Geometry check sheet. Reference: drawing and pictorial views, mm from the part's lowest x, y, z. A direction names the side the tool comes from. Round coordinates to 2 decimals unless told otherwise and drop trailing zeros. Write each loop counter-clockwise with the first axis right and the second up, starting at its lowest first coordinate (ties: lowest second). Pieces come first, ordered by that corner, then holes. Notation, with made-up numbers: M 68.25,75.25 L 99.25,75.25 A35 ccw 99.25,109.25 Z; hole C -32.5,-3 d5. An arc over 180 degrees is marked long. Use a Markdown table: item, result. Add a question column.
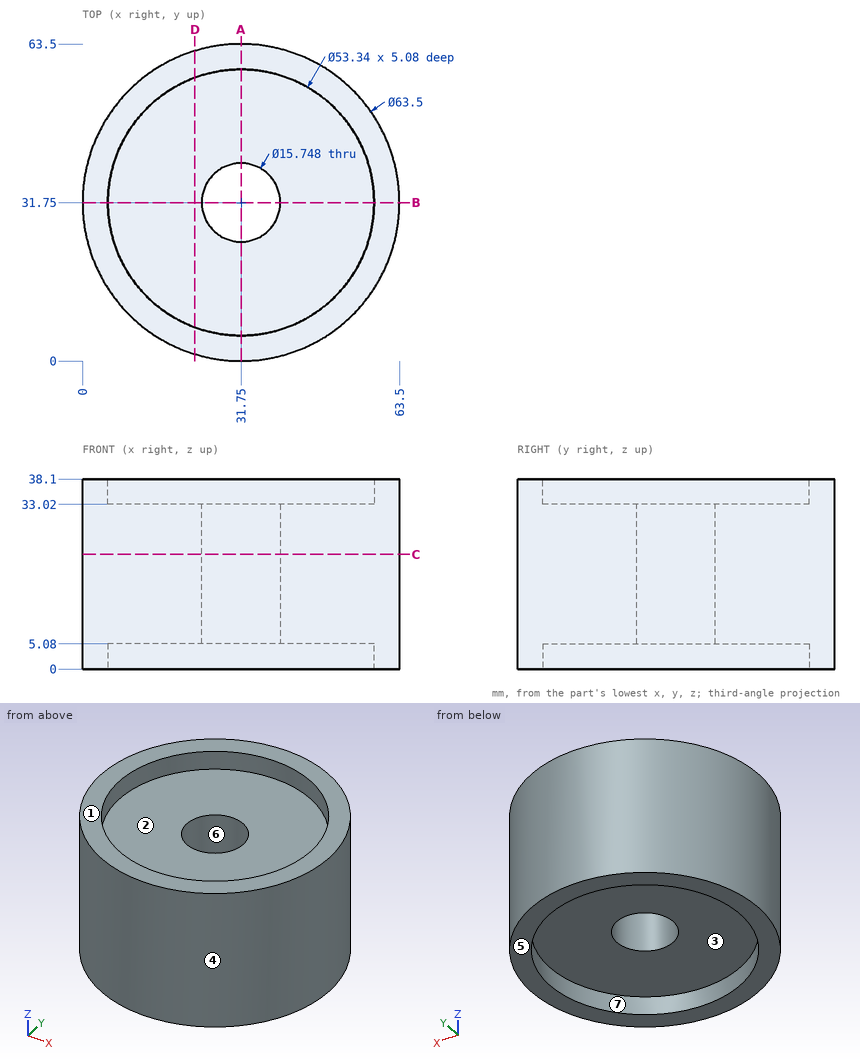
1. Access from +Z, -Z, +X, -X, +Y, -Y to the whole of each face (thin tool, end or side, straight path). Record for the marked faces 1, 2 and 3.
2. Scan lines: line 1 along Z through (x, y) = (30.5, 42.5); line 2 along Y through (x, z) = (31.75, 26); line 3 along X through (y, z) = (34, 22). Record each from-to range of solid material in increasing order. Write a range as from..to.
3. Cross-section at A-A on x = 31.75. Enter the section's corners in (y, z), plus the area to 3 significant figures.
4. Cross-section at C-C on z = 23. Enter the section's corners in (x, y).
5. Release check for a two-part mould opening along Y. For the marked faces 4, 5, 6 and 7 record: +Y half, -Y half, draft (parallel to the pull), parting line (faces both ways), or undercut.
6. Cross-section at D-D on x = 22.5. Enter the section's corners in (y, z).
7. Depth check by flat-ended pin: pin 1 Ø6 at (y, z) = (25.5, 4.5) entering from +X; pin 2 Ø5 at (x, z) = (29.5, 30.5) entering from +Y; pin 3 Ø2 at (y, z) = (15, 32) entering from +X. Enter the tip coordinate at first touch or a pass-through.
Answer:
| question | item | result |
|---|---|---|
| 1 | face 1 | +Z, +X, -X, +Y, -Y |
| 1 | face 2 | +Z |
| 1 | face 3 | -Z |
| 2 | line 1 | z = 5.08..33.02 |
| 2 | line 2 | y = 0..23.88, 39.62..63.5 |
| 2 | line 3 | x = 0.08..24.2, 39.3..63.42 |
| 3 | outline | M 0,0 L 5.08,0 L 5.08,5.08 L 23.88,5.08 L 23.88,33.02 L 5.08,33.02 L 5.08,38.1 L 0,38.1 Z; M 39.62,5.08 L 58.42,5.08 L 58.42,0 L 63.5,0 L 63.5,38.1 L 58.42,38.1 L 58.42,33.02 L 39.62,33.02 Z |
| 3 | area | 1,440 mm^2 |
| 4 | outline | C 31.75,31.75 d63.5; hole C 31.75,31.75 d15.75 |
| 5 | face 4 | parting line |
| 5 | face 5 | draft |
| 5 | face 6 | undercut |
| 5 | face 7 | undercut |
| 6 | outline | M 1.38,0 L 6.74,0 L 6.74,5.08 L 56.76,5.08 L 56.76,0 L 62.12,0 L 62.12,38.1 L 56.76,38.1 L 56.76,33.02 L 6.74,33.02 L 6.74,38.1 L 1.38,38.1 Z |
| 7 | pin 1 | stops at x = 63.33 |
| 7 | pin 2 | stops at y = 63.5 |
| 7 | pin 3 | stops at x = 59.32 |
